Could you check a few things on this model? Use its own coordinates, in mm. Give positions to 0.01 mm unless a question says otherwise; leave off trailing zeros. Write each loop counter-clockwise with the first axis right and the second up, starting at its lowest first coordinate (ties: lowest second). Pieces come first, ordered by that corner, then holes. Notation, with made-up numbers: (16.25, 57.5) - (26.25, 57.5) arc R15 cw to (26.25, 67.5) - close; hole circle Ø6 at (87, 19.5). An arc over 180 degrees is marked (long way). Answer in a Markdown table with one row per item.
from build123d import *

# Parameters (mm, degrees)
BOSS_EXTRUDE1_DEPTH = 4
SCALE1_SCALE        = 0.709677419


with BuildPart() as part:
    # Sketch1 → Boss-Extrude1 (new body)
    with BuildSketch(Plane.XY):
        with BuildLine():
            Line((150.379434294, 210.939689278), (158.72889788, 210.939689278))
            ThreePointArc((158.72889788, 210.939689278), (173.428975494, 206.161156043), (182.509468353, 193.652306729))
            Line((182.509468353, 193.652306729), (185.322557622, 184.978614816))
            ThreePointArc((185.322557622, 184.978614816), (184.66479187, 181.275668941), (181.2248759, 179.755326197))
            Line((181.2248759, 179.755326197), (151.16831456, 181.96131235))
            ThreePointArc((151.16831456, 181.96131235), (146.791215107, 183.665156491), (144.12485117, 187.532014108))
            Line((144.12485117, 187.532014108), (140.843128941, 197.929891907))
            ThreePointArc((140.843128941, 197.929891907), (142.314139082, 206.851627467), (150.379434294, 210.939689278))
        make_face()
    extrude(amount=BOSS_EXTRUDE1_DEPTH)


with BuildPart() as part_1:
    # Scale1: scaled about (162.020760572, 194.926645474, 2)
    add(part.part.scale(SCALE1_SCALE).moved(Location((47.038285327, 56.591606751, 0.580645161))))


solid = part_1.part
1) If I drill on line 1 (X direction, y = 200.25, z = 1.5); line 2 (X direction, y = 186.5, z = 1.65); line 3 (Y direction, x = 159, z = 2.1), over which ranges is the centre line in solid material (lowest first)?
Check values:
| item | result |
|---|---|
| line 1 | x = 146.74 to 173.02 |
| line 2 | x = 151.85 to 178.65 |
| line 3 | y = 185.38 to 206.29 |
2) Will these pins go through, and if not, where does the flat tip stop? P1, Ø1, axis at x = 173, z = 1, coming from the +Y side; P2, Ø1.5, axis at x = 168, z = 1.5, coming from the -Y side; P3, Ø1, axis at x = 153.5, z = 2.5, coming from the -Y side.
Check values:
| item | result |
|---|---|
| P1 | stops at y = 200.82 |
| P2 | stops at y = 184.67 |
| P3 | stops at y = 185.76 |
3) Imagine slicing it at B-B (x = 170). List the corners of the cut face in (y, z) for me, then the cut area to 3 significant figures.
Check values:
| item | result |
|---|---|
| outline | (184.57, 0.58) - (202.98, 0.58) - (202.98, 3.42) - (184.57, 3.42) - close |
| area | 52.3 mm2 |
4) Imagine slicing it at C-C (y = 187). List the corners of the cut face in (x, z) for me, then the cut area to 3 significant figures.
Check values:
| item | result |
|---|---|
| outline | (151.13, 0.58) - (178.7, 0.58) - (178.7, 3.42) - (151.13, 3.42) - close |
| area | 78.2 mm2 |
5) Imagine slicing it at A-A (z = 2.2). List the corners of the cut face in (x, y) for me, then the cut area to 3 significant figures.
Check values:
| item | result |
|---|---|
| outline | (146.99, 197.06) - (149.32, 189.68) arc R5.68 ccw to (154.32, 185.73) - (175.65, 184.16) arc R2.84 ccw to (178.56, 187.87) - (176.56, 194.02) arc R17.74 ccw to (159.68, 206.29) - (153.76, 206.29) arc R7.1 ccw to start |
| area | 552 mm2 |
